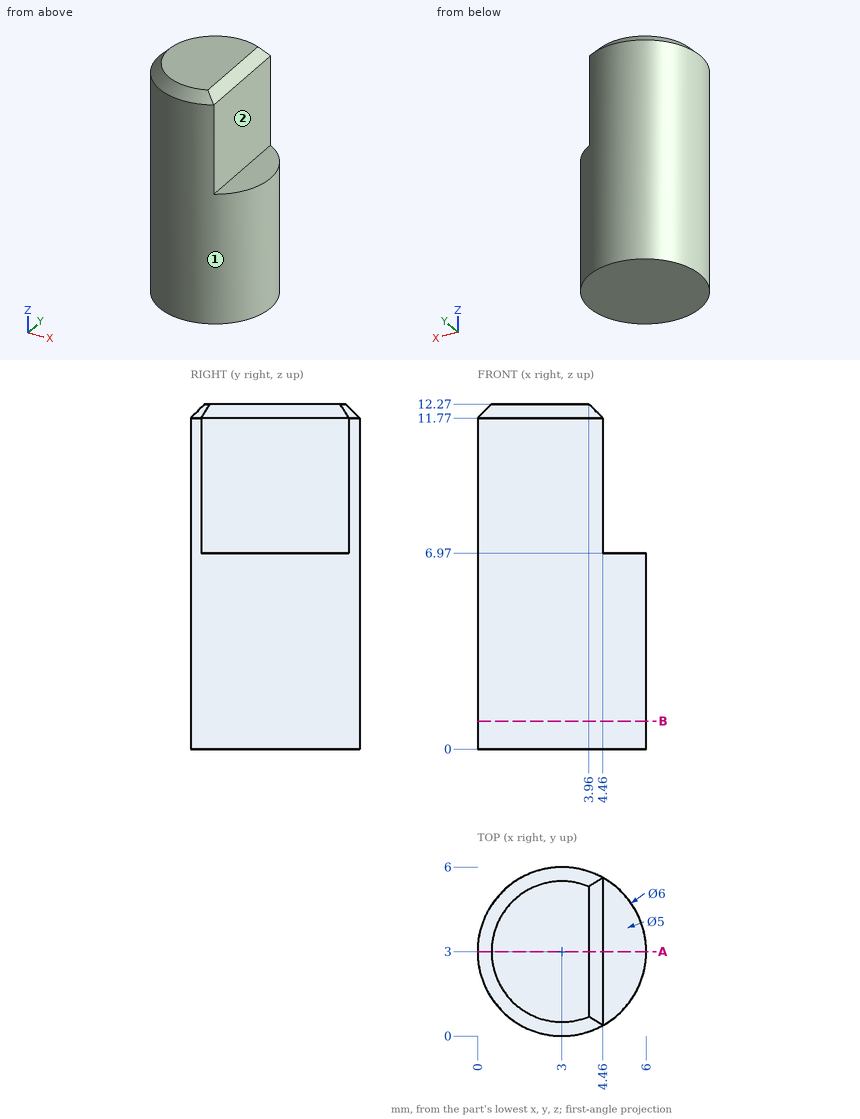
Could you check a few things on this drawing? It's one solid part, dimensions in mm from its lowest x, y, z. A direction names the side the tool comes from. Give positions to 0.01 mm unless a question says otherwise; leave off trailing zeros. Order: outer loops, then holes, each group sorted by start corner. A loop starts at its lowest first (then second) coordinate and runs counter-clockwise, first axis right, second up.
1. Suppose I cut it at A-A (y = 3). Write out the boundary of the cut face in (x, z), plus the area to 3 significant figures.
Answers below:
outline: (0, 0) - (6, 0) - (6, 6.97) - (4.46, 6.97) - (4.46, 11.77) - (3.96, 12.27) - (0.5, 12.27) - (0, 11.77) - close
area: 65.2 mm2
2. Suppose I cut it at B-B (z = 1). Write out the boundary of the cut face in (x, y), plus the area to 3 significant figures.
Answers below:
outline: circle Ø6 at (3, 3)
area: 28.3 mm2
3. Which directions (+Z, -Z, +X, -X, +Y, -Y) give clear straight access to the entire face, cutting with the end or side of a thin tool? Please do the marked faces 1 and 2.
Answers below:
face 1: +Z, -Z
face 2: +Z, +X, +Y, -Y
4. For pin 1 (0.8 mm diameter, centred on x = 5.5, y = 2.5, fed in from +Z); pin 2 (1.4 mm diameter, centred on y = 2, z = 8.5, fed in from +X), each with a flat end and sliding along its axis, tell me the tip position at first contact or that it passes through.
Answers below:
pin 1: stops at z = 6.97
pin 2: stops at x = 4.46
5. I need wall thicknesses on L1, parallel to Z at x = 4.5, y = 4.75; L2, parallel to X at y = 0.75, z = 10.75; L3, parallel to X at y = 4, z = 7.25. Which ranges of each line are inside material? Lowest first, please.
Answers below:
L1: z = 0 to 6.97
L2: x = 1.02 to 4.46
L3: x = 0.17 to 4.46
